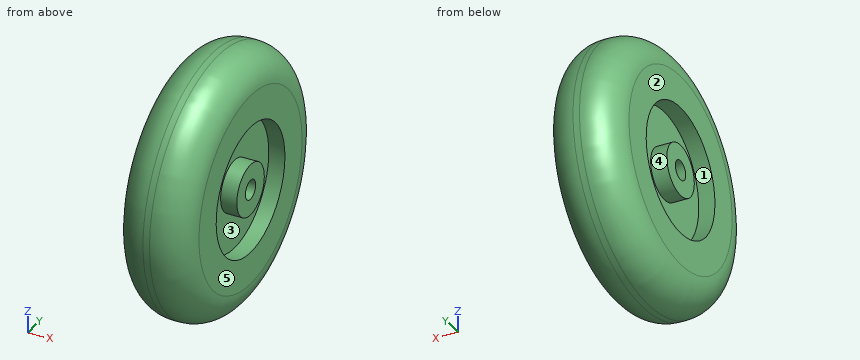
```python
from build123d import *

# Parameters (mm, degrees)
SKETCH2_R           = 20
SKETCH2_R_2         = 1.5
BOSS_EXTRUDE1_DEPTH = 5.5
FILLET1_R           = 5
SKETCH3_R           = 10
SKETCH3_R_2         = 4
CUT_EXTRUDE1_DEPTH  = 2.5
CUT_EXTRUDE2_START  = -2.5
SKETCH4_R           = 10
SKETCH4_R_2         = 4
CUT_EXTRUDE2_DEPTH  = 2.5


with BuildPart() as part:
    # Sketch2 → Boss-Extrude1 (new, symmetric)
    with BuildSketch(Plane(origin=(0, 0, 0), x_dir=(0, 0, -1), z_dir=(1, 0, 0))):
        Circle(SKETCH2_R)
        Circle(SKETCH2_R_2, mode=Mode.SUBTRACT)
    extrude(amount=BOSS_EXTRUDE1_DEPTH, both=True)

    # Fillet1
    fillet1_edges = [part.edges().sort_by_distance(p)[0] for p in [
        (-5.5, 0, 20),
        (5.5, 0, 20),
    ]]
    fillet(fillet1_edges, radius=FILLET1_R)

    # Sketch3 → Cut-Extrude1 (cut)
    with BuildSketch(Plane(origin=(5.5, 0, 0), x_dir=(0, 0, -1), z_dir=(1, 0, 0))):
        Circle(SKETCH3_R)
        Circle(SKETCH3_R_2, mode=Mode.SUBTRACT)
    extrude(amount=-CUT_EXTRUDE1_DEPTH, mode=Mode.SUBTRACT)

    # Sketch4 → Cut-Extrude2 (cut)
    with BuildSketch(Plane.ZY.offset(5.5).offset(CUT_EXTRUDE2_START)):
        with Locations(Location((0, 0, 0), (0, 0, 180))):
            Circle(SKETCH4_R)
        with Locations(Location((0, 0, 0), (0, 0, 180))):
            Circle(SKETCH4_R_2, mode=Mode.SUBTRACT)
    extrude(amount=CUT_EXTRUDE2_DEPTH, mode=Mode.SUBTRACT)


solid = part.part
```
Source: CAD feature listing. Evaluate the final solid. Frame: model axes, mm. Face numbers are marked on the shaded views. A direction names the side the tool comes from. Coordinates: 2 decimals unless noted, no trailing zeros. Loops run counter-clockwise (first coordinate to the right, second up) from the corner with the lowest first, then second, coordinate; pieces in that order, holes last. Notation, with made-up numbers: (20.25, 73) -> (25.25, 73) arc R24 ccw to (25.25, 84) -> close; hole circle Ø4 at (57, 39.5). An arc over 180 degrees is marked (long way). One line per item, written item: value. Start each with the question number.
Q1. Section query A-A, the plane y = 0. Return the cut outline in (x, z).
Q2. Section query C-C, the plane x = -4.5. Return the cut outline in (y, z).
Q3. Set-up query: the marked faces 1, 2 and 3. Return all of +Z, -Z, +X, -X, +Y, -Y with unobstructed straight access to the full face (end or side cutting, diameter ignored); none if empty.
Q4. Section query D-D, the plane x = 0. Return the cut outline in (y, z), and give its area (3 significant figures).
Q5. Contact query for flat-ended pins moving along their axis: P1, Ø3, axis at y = 14.5, z = 9, coming from the -X side; P2, Ø3, axis at x = 3.5, y = 6.5, coming from the +Z side; P3, Ø5, axis at x = -4, y = 6.5, coming from the -Z side. Output: stop coordinate, or through.
Q6. Line query: line 1 along Y through (x, z) = (3.5, -3); line 2 along X through (y, z) = (6, 1); line 3 along Y through (x, z) = (4, -2.5). Output: solid intervals per line, ascending.
Q7. Mould query, pull axis Y, two halves, no side actions, for the marked faces 4 and 5. Classes: pulls with the +Y half, pulls with the -Y half, needs draft (parallel to the pull), parting line crosses it, or undercut.
Results:
1. outline: (-5.5, -15) arc R5 ccw to (-0.5, -20) -> (0.5, -20) arc R5 ccw to (5.5, -15) -> (5.5, -10) -> (3, -10) -> (3, -4) -> (5.5, -4) -> (5.5, -1.5) -> (-5.5, -1.5) -> (-5.5, -4) -> (-3, -4) -> (-3, -10) -> (-5.5, -10) -> close; (-5.5, 1.5) -> (5.5, 1.5) -> (5.5, 4) -> (3, 4) -> (3, 10) -> (5.5, 10) -> (5.5, 15) arc R5 ccw to (0.5, 20) -> (-0.5, 20) arc R5 ccw to (-5.5, 15) -> (-5.5, 10) -> (-3, 10) -> (-3, 4) -> (-5.5, 4) -> close
2. outline: circle Ø36 at (0, 0); circle Ø8 at (0, 0); hole circle Ø20 at (0, 0); hole circle Ø3 at (0, 0)
3. face 1: -X
3. face 2: +Z, -Z, -X, +Y, -Y
3. face 3: +X
4. outline: circle Ø40 at (0, 0); hole circle Ø3 at (0, 0)
4. area: 1,250 mm^2
5. P1: x = -5.47
5. P2: z = 18.85
5. P3: z = -19.13
6. line 1: -18.76 to -9.54, -2.65 to 2.65, 9.54 to 18.76
6. line 2: -3 to 3
6. line 3: -18.4 to -9.68, -3.12 to 3.12, 9.68 to 18.4
7. face 4: undercut
7. face 5: needs draft
